```python
from build123d import *

# Parameters (mm, degrees)
SKETCH1_R           = 21
SKETCH1_R_2         = 5
SKETCH1_R_3         = 2
BOSS_EXTRUDE1_DEPTH = 8
BOSS_EXTRUDE2_START = 4
SKETCH1_3_R         = 21
SKETCH1_3_R_2       = 19
BOSS_EXTRUDE2_DEPTH = 4
SKETCH1_4_R         = 21
SKETCH1_4_R_2       = 19
SKETCH1_4_R_3       = 15
BOSS_EXTRUDE3_DEPTH = 12
SKETCH1_6_R         = 5
SKETCH1_6_R_2       = 2
BOSS_EXTRUDE4_DEPTH = 4
BOSS_EXTRUDE5_START = 4
SKETCH1_7_R         = 5
SKETCH1_7_R_2       = 2
BOSS_EXTRUDE5_DEPTH = 4
SKETCH1_8_R         = 5
SKETCH1_8_R_2       = 2
BOSS_EXTRUDE6_DEPTH = 8


with BuildPart() as part:
    # Sketch1 → Boss-Extrude1 (new body)
    with BuildSketch(Plane.XY):
        Circle(SKETCH1_R)
        Circle(SKETCH1_R_2, mode=Mode.SUBTRACT)
        with Locations((0, 12)):
            Circle(SKETCH1_R_3, mode=Mode.SUBTRACT)
        with Locations((10.392304845, 6)):
            Circle(SKETCH1_R_3, mode=Mode.SUBTRACT)
        with Locations((10.392304845, -6)):
            Circle(SKETCH1_R_3, mode=Mode.SUBTRACT)
        with Locations((0, -12)):
            Circle(SKETCH1_R_3, mode=Mode.SUBTRACT)
        with Locations((-10.392304845, -6)):
            Circle(SKETCH1_R_3, mode=Mode.SUBTRACT)
        with Locations((-10.392304845, 6)):
            Circle(SKETCH1_R_3, mode=Mode.SUBTRACT)
    extrude(amount=-BOSS_EXTRUDE1_DEPTH)

    # Sketch1<3> → Boss-Extrude2 (add)
    with BuildSketch(Plane.XY.offset(BOSS_EXTRUDE2_START)):
        Circle(SKETCH1_3_R)
        Circle(SKETCH1_3_R_2, mode=Mode.SUBTRACT)
    extrude(amount=-BOSS_EXTRUDE2_DEPTH)

    # Sketch1<4> → Boss-Extrude3 (add)
    # profile 1 of 2: a face of its own
    with BuildSketch(Plane.XY):
        Circle(SKETCH1_4_R)
        Circle(SKETCH1_4_R_2, mode=Mode.SUBTRACT)
    # profile 2 of 2: a face of its own
    with BuildSketch(Plane.XY):
        Circle(SKETCH1_4_R_2)
        Circle(SKETCH1_4_R_3, mode=Mode.SUBTRACT)
    extrude(amount=-BOSS_EXTRUDE3_DEPTH)



with BuildPart() as body_2:
    # Sketch1<6> → Boss-Extrude4 (new body)
    with BuildSketch(Plane.XY):
        Circle(SKETCH1_6_R)
        Circle(SKETCH1_6_R_2, mode=Mode.SUBTRACT)
    extrude(amount=BOSS_EXTRUDE4_DEPTH)

    # Sketch1<7> → Boss-Extrude5 (add)
    with BuildSketch(Plane.XY.offset(BOSS_EXTRUDE5_START)):
        Circle(SKETCH1_7_R)
        Circle(SKETCH1_7_R_2, mode=Mode.SUBTRACT)
    extrude(amount=-BOSS_EXTRUDE5_DEPTH)


with BuildPart() as part_1:
    add(part.part)

    add(body_2.part)  # Boss-Extrude6 merges body 2
    # Sketch1<8> → Boss-Extrude6 (add)
    with BuildSketch(Plane.XY):
        Circle(SKETCH1_8_R)
        Circle(SKETCH1_8_R_2, mode=Mode.SUBTRACT)
    extrude(amount=-BOSS_EXTRUDE6_DEPTH)


solid = part_1.part
```
Source: CAD feature listing. Evaluate the final solid. Frame: model axes, mm. A direction names the side the tool comes from. Give positions to 0.01 mm unless a question says otherwise; leave off trailing zeros. Write each loop counter-clockwise with the first axis right and the second up, starting at its lowest first coordinate (ties: lowest second). Pieces come first, ordered by that corner, then holes. Notation, with made-up numbers: (-24.75, -7.75) - (1.25, -7.75) arc R22 ccw to (1.25, 12.25) - close; hole circle Ø10 at (-31, 18). An arc over 180 degrees is marked (long way). One line per item, written item: value. Start each with the question number.
Q1. Section query C-C, the plane z = -5.75. Return the cut outline in (x, y).
Q2. Section query B-B, the plane x = 0. Return the cut outline in (y, z).
Q3. Section query A-A, the plane y = 0. Return the cut outline in (x, z), then the cut area to 3 significant figures.
Q4. Section query D-D, the plane x = 10.5. Return the cut outline in (y, z), then the cut area to 3 significant figures.
Q5. Draft query along X for faces 4 (the face through (20.03, 6.31, -3.89)), 5 (the face through (-16, -11, 4)), 6 (the face through (4, -4, 0)). Return one class per face: +X half, -X half, draft (parallel to the pull), parting line (faces both ways), or undercut.
Q6. First-contact query: pin 1 Ø2.5 at (x, y) = (0, 0) entering from +Z; pin 2 Ø11 at (x, y) = (-0.5, -1) entering from -Z; pin 3 Ø6 at (x, z) = (-9.5, 0.5) entering from -Y; pin 4 Ø4.5 at (x, y) = (-10.39, 6) entering from +Z. Flat tips, straight axial feed; report the tip coordinate or a pass-through.
Q7. Material intervals for probe 1 along Y at (x, z) = (11, -3); probe 2 along Z at (x, y) = (-8, 13.5); probe 3 along Y at (x, z) = (-9, -5.5), sorted ascending. Write a range as from..to.
Q8. Set-up query: faces 1 (the face through (8.767, -16.856, 2.028)), 2 (the face through (-14.985, 0.66, -9.972)), 3 (the face through (8.394, -5.912, -3.944)). Return all of +Z, -Z, +X, -X, +Y, -Y with unobstructed straight access to the full face (end or side cutting, diameter ignored); none if empty.
Answer:
1. outline: circle Ø42 at (0, 0); hole circle Ø4 at (-10.39, -6); hole circle Ø4 at (-10.39, 6); hole circle Ø4 at (0, -12); hole circle Ø4 at (0, 0); hole circle Ø4 at (0, 12); hole circle Ø4 at (10.39, -6); hole circle Ø4 at (10.39, 6)
2. outline: (-21, -12) - (-15, -12) - (-15, -8) - (-14, -8) - (-14, 0) - (-19, 0) - (-19, 4) - (-21, 4) - close; (-10, -8) - (-2, -8) - (-2, 4) - (-5, 4) - (-5, 0) - (-10, 0) - close; (2, -8) - (10, -8) - (10, 0) - (5, 0) - (5, 4) - (2, 4) - close; (14, -8) - (15, -8) - (15, -12) - (21, -12) - (21, 4) - (19, 4) - (19, 0) - (14, 0) - close
3. outline: (-21, -12) - (-15, -12) - (-15, -8) - (-2, -8) - (-2, 4) - (-5, 4) - (-5, 0) - (-19, 0) - (-19, 4) - (-21, 4) - close; (2, -8) - (15, -8) - (15, -12) - (21, -12) - (21, 4) - (19, 4) - (19, 0) - (5, 0) - (5, 4) - (2, 4) - close
3. area: 392 mm2
4. outline: (-18.19, -12) - (-10.71, -12) - (-10.71, -8) - (-8, -8) - (-8, 0) - (-15.84, 0) - (-15.84, 4) - (-18.19, 4) - close; (-4, -8) - (4, -8) - (4, 0) - (-4, 0) - close; (8, -8) - (10.71, -8) - (10.71, -12) - (18.19, -12) - (18.19, 4) - (15.84, 4) - (15.84, 0) - (8, 0) - close
4. area: 306 mm2
5. face 4: parting line
5. face 5: draft
5. face 6: undercut
6. pin 1: passes through
6. pin 2: stops at z = -8
6. pin 3: stops at y = -19.97
6. pin 4: stops at z = 0
7. probe 1: y = -17.89..-7.91, -4.09..4.09, 7.91..17.89
7. probe 2: z = -12..0
7. probe 3: y = -18.97..-7.44, -4.56..4.56, 7.44..18.97
8. face 1: +Z
8. face 2: -Z
8. face 3: +Z, -Z
